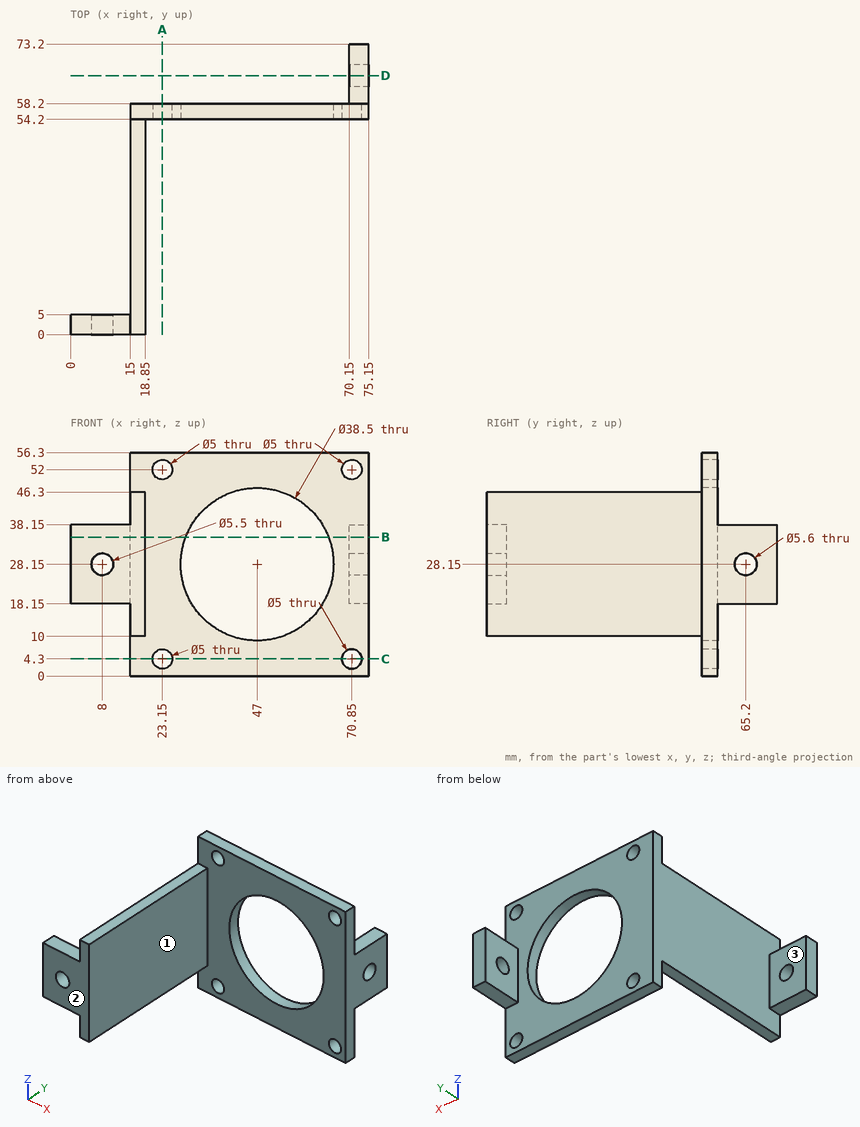
Check sheet for the drawn part. Datum: minimum x, y, z corner. Units: mm. A direction names the side the tool comes from. Round coordinates to 2 decimals unless told otherwise and drop trailing zeros. Loops run counter-clockwise (first coordinate to the right, second up) from the corner with the lowest first, then second, coordinate; pieces in that order, holes last. Notation, with made-up numbers: (-2, 82) - (56, 82) arc R35 cw to (56, 116) - close; hole circle Ø3 at (73.5, -16). An arc over 180 degrees is marked (long way). Write each question's results on one line, items separated by ' | '. Start each with the question number.
Q1. Cross-section at A-A on x = 23.15. Enter the section's corners in (y, z), and give its area (3 significant figures).
Q2. Cross-section at D-D on y = 65.2. Enter the section's corners in (x, z), and give its area (3 significant figures).
Q3. Gauge pin test, flat ends, axial feed: P1, Ø4.5, axis at x = 10.5, z = 26.5, coming from the +Y side; P2, Ø6, axis at y = 18, z = 47, coming from the +X side; P3, Ø10, axis at y = 57.5, z = 47, coming from the -X side; P4, Ø6, axis at x = 11, z = 19.5, coming from the -Y side. Record the tip position at first contact, or that the pin passes through.
Q4. Cross-section at B-B on z = 35. Enter the section's corners in (x, y).
Q5. Access from +Z, -Z, +X, -X, +Y, -Y to the whole of each face (thin tool, end or side, straight path). Record for the marked faces 1, 2 and 3.
Q6. Cross-section at C-C on z = 4.3. Enter the section's corners in (x, y).
Q7. Thickness scan on line 1 (Z direction, x = 23.15, y = 57.3); line 2 (X direction, y = 55, z = 52); line 3 (Z direction, x = 47, y = 55). Record the ranges inside material, lowest first. Write a range as [from, to].
Answers below:
1) outline: (54.2, 0) - (58.2, 0) - (58.2, 1.8) - (54.2, 1.8) - close; (54.2, 6.8) - (58.2, 6.8) - (58.2, 49.5) - (54.2, 49.5) - close; (54.2, 54.5) - (58.2, 54.5) - (58.2, 56.3) - (54.2, 56.3) - close | area: 185 mm²
2) outline: (70.15, 18.15) - (75.15, 18.15) - (75.15, 25.35) - (70.15, 25.35) - close; (70.15, 30.95) - (75.15, 30.95) - (75.15, 38.15) - (70.15, 38.15) - close | area: 72.0 mm²
3) P1: stops at y = 5 | P2: stops at x = 18.85 | P3: stops at x = 15 | P4: stops at y = 0
4) outline: (0, 0) - (18.85, 0) - (18.85, 54.2) - (29.01, 54.2) - (29.01, 58.2) - (15, 58.2) - (15, 5) - (0, 5) - close; (64.99, 54.2) - (75.15, 54.2) - (75.15, 73.2) - (70.15, 73.2) - (70.15, 58.2) - (64.99, 58.2) - close
5) face 1: +Z, -Z, +X, -Y | face 2: +Z, -Z, +X, -X, -Y | face 3: +Z, -Z, -X, +Y
6) outline: (15, 54.2) - (20.65, 54.2) - (20.65, 58.2) - (15, 58.2) - close; (25.65, 54.2) - (68.35, 54.2) - (68.35, 58.2) - (25.65, 58.2) - close; (73.35, 54.2) - (75.15, 54.2) - (75.15, 58.2) - (73.35, 58.2) - close
7) line 1: z = [0, 1.8], [6.8, 49.5], [54.5, 56.3] | line 2: x = [15, 20.65], [25.65, 68.35], [73.35, 75.15] | line 3: z = [0, 8.9], [47.4, 56.3]
